Geometry: final body of the model. Coordinates: model frame, mm. A direction names the side the tool comes from. Round coordinates to 2 decimals unless told otherwise and drop trailing zeros. Write each loop counter-clockwise with the first axis right and the second up, starting at its lowest first coordinate (ties: lowest second). Pieces come first, ordered by that corner, then holes. Notation, with made-up numbers: M 70.5,3 L 75.5,3 A27 ccw 75.5,29 Z; hole C 41.25,83 d3. An arc over 180 degrees is marked long. Use one line per item in the form item = value. Start each with the question number.
from build123d import *

# Parameters (mm, degrees)
SKETCH1_W              = 185.4
SKETCH1_H              = 190
BASE_PLATE_DEPTH       = 6.35
SLOTS_DEPTH            = 7.35
FEET_CONNECTION_HOLE_D = 6.7564


with BuildPart() as part:
    # Sketch1 → base plate (new body)
    with BuildSketch(Plane(origin=(0, 0, 0), x_dir=(1, 0, 0), z_dir=(0, 1, 0))):
        with Locations((92.7, -95)):
            Rectangle(SKETCH1_W, SKETCH1_H)
    extrude(amount=-BASE_PLATE_DEPTH)

    # Sketch3 → slots (cut, through all)
    with BuildSketch(Plane(origin=(0, 0, 0), x_dir=(1, 0, 0), z_dir=(0, 1, 0))):
        with BuildLine():
            ThreePointArc((21.424612456, -27.64618524), (21.424612456, -30.474612456), (18.59618524, -30.474612456))
            Line((18.59618524, -30.474612456), (13.208031568, -25.086458783))
            ThreePointArc((13.208031568, -25.086458783), (13.208031568, -22.258031568), (16.036458783, -22.258031568))
            Line((16.036458783, -22.258031568), (21.424612456, -27.64618524))
        make_face()
        with BuildLine():
            Line((169.363541217, -22.258031568), (163.975387544, -27.64618524))
            ThreePointArc((163.975387544, -27.64618524), (163.975387544, -30.474612456), (166.80381476, -30.474612456))
            Line((166.80381476, -30.474612456), (172.191968432, -25.086458783))
            ThreePointArc((172.191968432, -25.086458783), (172.191968432, -22.258031568), (169.363541217, -22.258031568))
        make_face()
        with BuildLine():
            Line((154.995131423, -42.283295792), (160.383285096, -36.895142119))
            ThreePointArc((160.383285096, -36.895142119), (160.383285096, -34.066714904), (157.554857881, -34.066714904))
            Line((157.554857881, -34.066714904), (152.166704208, -39.454868577))
            ThreePointArc((152.166704208, -39.454868577), (152.166704208, -42.283295792), (154.995131423, -42.283295792))
        make_face()
        with BuildLine():
            ThreePointArc((160.383285096, -153.104857881), (160.383285096, -155.933285096), (157.554857881, -155.933285096))
            Line((157.554857881, -155.933285096), (152.166704208, -150.545131423))
            ThreePointArc((152.166704208, -150.545131423), (152.166704208, -147.716704208), (154.995131423, -147.716704208))
            Line((154.995131423, -147.716704208), (160.383285096, -153.104857881))
        make_face()
        with BuildLine():
            ThreePointArc((163.975387544, -162.35381476), (163.975387544, -159.525387544), (166.80381476, -159.525387544))
            Line((166.80381476, -159.525387544), (172.191968432, -164.913541217))
            ThreePointArc((172.191968432, -164.913541217), (172.191968432, -167.741968432), (169.363541217, -167.741968432))
            Line((169.363541217, -167.741968432), (163.975387544, -162.35381476))
        make_face()
        with BuildLine():
            Line((16.036458783, -167.741968432), (21.424612456, -162.35381476))
            ThreePointArc((21.424612456, -162.35381476), (21.424612456, -159.525387544), (18.59618524, -159.525387544))
            Line((18.59618524, -159.525387544), (13.208031568, -164.913541217))
            ThreePointArc((13.208031568, -164.913541217), (13.208031568, -167.741968432), (16.036458783, -167.741968432))
        make_face()
        with BuildLine():
            Line((30.404868577, -147.716704208), (25.016714904, -153.104857881))
            ThreePointArc((25.016714904, -153.104857881), (25.016714904, -155.933285096), (27.845142119, -155.933285096))
            Line((27.845142119, -155.933285096), (33.233295792, -150.545131423))
            ThreePointArc((33.233295792, -150.545131423), (33.233295792, -147.716704208), (30.404868577, -147.716704208))
        make_face()
        with BuildLine():
            Line((30.404868577, -42.283295792), (25.016714904, -36.895142119))
            ThreePointArc((25.016714904, -36.895142119), (25.016714904, -34.066714904), (27.845142119, -34.066714904))
            Line((27.845142119, -34.066714904), (33.233295792, -39.454868577))
            ThreePointArc((33.233295792, -39.454868577), (33.233295792, -42.283295792), (30.404868577, -42.283295792))
        make_face()
    extrude(amount=-SLOTS_DEPTH, mode=Mode.SUBTRACT)

    # Feet connection hole (through all)
    with Locations(Plane(origin=(0, 0, 0), x_dir=(1, 0, 0), z_dir=(0, 1, 0))):
        with Locations((47.7, -177.3), (137.7, -12.7), (47.7, -12.7), (137.7, -177.3)):
            Hole(FEET_CONNECTION_HOLE_D / 2)


solid = part.part
1. Ray query, probe 1 along X at (y, z) = (-3.75, 177.3); probe 2 along Z at (x, y) = (137.7, -4.75); probe 3 along Z at (x, y) = (20, -3.5). Return the intervals inside material, ascending.
2. Pull-direction query (Z, two-part tool) for faces 3 (the face through (91, -3, 0)), 4 (the face through (91, 0, 94)), 5 (the face through (48.14, -3.22, 173.95)); classes: released by +Z, released by -Z, zero draft, split by the parting line, or undercut.
3. Set-up query: faces 1 (the face through (91, -6.35, 94)), 2 (the face through (154.9, -3.13, 153.28)). Return all of +Z, -Z, +X, -X, +Y, -Y with unobstructed straight access to the full face (end or side cutting, diameter ignored); none if empty.
4. Contact query for flat-ended pins moving along their axis: pin 1 (2 mm diameter, centred on x = 108, y = -4, fed in from -Z); pin 2 (5.5 mm diameter, centred on x = 47.7, z = 177.3, fed in from +Y). Output: stop coordinate, or through.
5. Section query A-A (z = 12.7). Return loops of the section in (x, y).
6. Section query B-B (x = 47.7). Return loops of the section in (y, z), then the cut area to 3 significant figures.
Checks:
q1.probe_1 = 0 to 44.32, 51.08 to 134.32, 141.08 to 185.4
q1.probe_2 = 0 to 9.32, 16.08 to 173.92, 180.68 to 190
q1.probe_3 = 0 to 26.22, 31.06 to 158.94, 163.78 to 190
q2.face_3 = released by -Z
q2.face_4 = zero draft
q2.face_5 = undercut
q3.face_1 = +Z, -Z, +X, -X, -Y
q3.face_2 = +Y, -Y
q4.pin_1 = 0
q4.pin_2 = through
q5.outline = M 0,-6.35 L 44.32,-6.35 L 44.32,0 L 0,0 Z; M 51.08,-6.35 L 134.32,-6.35 L 134.32,0 L 51.08,0 Z; M 141.08,-6.35 L 185.4,-6.35 L 185.4,0 L 141.08,0 Z
q6.outline = M -6.35,0 L 0,0 L 0,9.32 L -6.35,9.32 Z; M -6.35,16.08 L 0,16.08 L 0,173.92 L -6.35,173.92 Z; M -6.35,180.68 L 0,180.68 L 0,190 L -6.35,190 Z
q6.area = 1,120 mm^2
